The model under review builds one solid part; all positions refer to its coordinate system, in mm. A direction names the side the tool comes from. Give positions to 0.01 mm unless a question says otherwise; leave off trailing zeros. Loops run counter-clockwise (first coordinate to the right, second up) from the corner with the lowest first, then second, coordinate; pieces in that order, holes last. Notation, with made-up numbers: M 22.5,-28 L 27.5,-28 A30 cw 27.5,10 Z; hole C 70.25,-31.75 d4. An arc over 180 degrees is marked long. Write item = value, one per line. Start each with the question number.
1. For faces 1 (the face through (140, 10, 6)), 2 (the face through (70, 1, 9)), 3 (the face through (130, 19, 9)), 4 (the face through (101, 20, 4)), list the 3-axis set-ups (+Z, -Z, +X, -X, +Y, -Y) from which the entire face can be reached by the end or side of a thin tool; tool diameter is ignored.
2. We need section C-C on y = 18. Give the boundary of the cut face in (x, z).
3. We need section D-D on x = 81.5. Give the boundary of the cut face in (y, z).
4. Draft analysis for pull direction X (two halves, no side actions). For faces 5 (the face through (168, 5, 5)), 6 (the face through (195, 10, 5)), 7 (the face through (2.255, 17.861, 5.07)), 8 (the face through (99, 0, 4)), state which applies: pulls with the +X half, pulls with the -X half, needs draft (parallel to the pull), parting line crosses it, or undercut.
5. Wall thickness on line 1 along X through (y, z) = (11.5, 1.25); line 2 along X through (y, z) = (5.25, 3); line 3 along Y through (x, z) = (39.5, 6.5): over which ranges is each line inside the solid? List them lowest first. Write a range as from..to.
6. We need section B-B on x = 148. Give the boundary of the cut face in (y, z).
7. We need section A-A on z = 3.25. Give the boundary of the cut face in (x, y), then the cut area to 3 significant figures.
8. For pin 1 (5.5 mm diameter, centred on y = 18.5, z = 7, fed in from +X); pin 2 (4 mm diameter, centred on y = 3, z = 8.5, fed in from -X); pin 3 (6 mm diameter, centred on x = 166.5, z = 3.5, fed in from -Y); pin 4 (2 mm diameter, centred on y = 15, z = 6.5, fed in from +X), all flat-tipped, find the tip position at first contact; note any pin that passes through.
Autodesk Fusion 360 part; units mm, degrees
sketch "Sketch1" plane through (0, 0, 0) normal (0, 0, 1) x (1, 0, 0)
  line L0 (0, 0) -> (200, 0)
  line L1 (200, 0) -> (200, 20)
  line L2 (200, 20) -> (0, 20)
  line L3 (0, 20) -> (0, 0)
  line L4 (100, 20) -> (130, 20)
  line L5 (130, 20) -> (130, 0)
  line L6 (130, 0) -> (100, 0)
  line L7 (100, 0) -> (100, 20)
  line L8 (130, 0) -> (70, 0)
  line L9 (70, 0) -> (70, 20)
  line L10 (70, 20) -> (130, 20)
  line L11 (130, 20) -> (130, 0)
  line L12 (140, 15) -> (195, 15)
  line L13 (195, 15) -> (195, 5)
  line L14 (195, 5) -> (140, 5)
  line L15 (140, 5) -> (140, 15)
  line L16 (60, 5) -> (5, 5)
  line L17 (5, 5) -> (5, 15)
  line L18 (5, 15) -> (60, 15)
  line L19 (60, 15) -> (60, 5)
  dimension "d1" = 200
  dimension "d2" = 20
extrude "Extrude1" add sketch "Sketch1" along normal blind 10
fillet "Fillet1" radius 7.5 4 edges at (200, 20, 5) (200, 0, 5) (0, 0, 5) (0, 20, 5)
sketch "Sketch2" plane through (0, 0, 10) normal (0, 0, 1) x (-1, 0, 0)
  arc A0 (-7.5, -20) -> (0, -12.5) centre (-7.5, -12.5) ccw
  line L0 (0, -12.5) -> (0, -7.5)
  arc A1 (0, -7.5) -> (-7.5, 0) centre (-7.5, -7.5) ccw
  line L1 (-7.5, 0) -> (-192.5, 0)
  arc A2 (-192.5, 0) -> (-200, -7.5) centre (-192.5, -7.5) ccw
  line L2 (-200, -7.5) -> (-200, -12.5)
  arc A3 (-200, -12.5) -> (-192.5, -20) centre (-192.5, -12.5) ccw
  line L3 (-192.5, -20) -> (-7.5, -20)
  line L4 (-195, -5) -> (-140, -5)
  line L5 (-140, -5) -> (-140, -15)
  line L6 (-140, -15) -> (-195, -15)
  line L7 (-195, -15) -> (-195, -5)
  line L8 (-5, -15) -> (-60, -15)
  line L9 (-60, -15) -> (-60, -5)
  line L10 (-60, -5) -> (-5, -5)
  line L11 (-5, -5) -> (-5, -15)
  line L12 (-60, -20) -> (-140, -20)
  line L13 (-140, -20) -> (-140, 0)
  line L14 (-140, 0) -> (-60, 0)
  line L15 (-60, 0) -> (-60, -20)
extrude "Extrude2" add sketch "Sketch2" along normal blind 2 contours L1 L3 L5 L9 L12 L13 L14 L15
extrude "Extrude3" cut 2 faces at (24.1667, 3.3333, 10) (175.8333, 3.3333, 10) along direction (0, 0, -1) blind 10
chamfer "Chamfer1" distance 7 angle 45 2 edges at (100, 0, 12) (100, 20, 12)
extrude "Extrude4" add sketch "Sketch1" along normal blind 10 contours L0 L2 L3 L9 | L0 L1 L2 L5 L11
fillet "Fillet2" radius 7.5 4 edges at (0, 20, 5) (0, 0, 5) (200, 20, 5) (200, 0, 5)
Final values:
q1.face_1 = +Z, -Z
q1.face_2 = +Z, -Y
q1.face_3 = +Z, +Y
q1.face_4 = +Z, -Z, +X, -X, +Y
q2.outline = M 2.4,0 L 197.6,0 L 197.6,10 L 130,10 L 130,7 L 70,7 L 70,10 L 2.4,10 Z
q3.outline = M 0,0 L 20,0 L 20,5 L 13,12 L 7,12 L 0,5 Z
q4.face_5 = undercut
q4.face_6 = undercut
q4.face_7 = pulls with the -X half
q4.face_8 = needs draft
q5.line_1 = 0..5, 60..140, 195..200
q5.line_2 = 0.35..5, 60..140, 195..199.65
q5.line_3 = 0..5, 15..20
q6.outline = M 0,0 L 5,0 L 5,10 L 0,10 Z; M 15,0 L 20,0 L 20,10 L 15,10 Z
q7.outline = M 0,7.5 A7.5 ccw 7.5,0 L 192.5,0 A7.5 ccw 200,7.5 L 200,12.5 A7.5 ccw 192.5,20 L 7.5,20 A7.5 ccw 0,12.5 Z; hole M 5,5 L 60,5 L 60,15 L 5,15 Z; hole M 140,5 L 195,5 L 195,15 L 140,15 Z
q7.area = 2,850 mm²
q8.pin_1 = 199.26
q8.pin_2 = 0.43
q8.pin_3 = 0
q8.pin_4 = 199.85
